from build123d import *

# Parameters (mm, degrees)
F0_W      = 100
F0_H      = 100
F1_DEPTH  = 20
F2_W      = 100
F2_H      = 20
F3_DEPTH  = 80
F4_W      = 30
F4_H      = 80
F5_DEPTH  = 80
F6_SIZE2  = 80
F6_SIZE   = 80
F7_W      = 15
F7_H      = 12.7048021555
F8_DEPTH  = 127
F10_DEPTH = 1143
F11_R     = 15.2311965997
F12_DEPTH = 254
F13_R     = 19.0095175901


with BuildPart() as f1:
    # F0 (on Front) → F1 (new body)
    with BuildSketch(Plane.XZ):
        Rectangle(F0_W, F0_H)
    extrude(amount=F1_DEPTH)

    # F2 (on face) → F3 (join)
    with BuildSketch(Plane.XZ.offset(20)):
        with Locations((0, 40)):
            Rectangle(F2_W, F2_H)
    extrude(amount=F3_DEPTH)

    # F4 (on face) → F5 (join)
    with BuildSketch(Plane.XZ.offset(20)):
        with Locations((35, -10)):
            Rectangle(F4_W, F4_H)
    extrude(amount=F5_DEPTH)

    # F6
    f6_edges = [f1.edges().sort_by_distance(p)[0] for p in [
        (35, -100, -50),
    ]]
    chamfer(f6_edges, length=F6_SIZE, length2=F6_SIZE2)

    # F7 (on face) → F8 (cut)
    with BuildSketch(Plane(origin=(0, 0, 30), x_dir=(1, 0, 0), z_dir=(0, 0, -1))):
        with Locations((-22.5, 66.3524010777)):
            Rectangle(F7_W, F7_H)
        with Locations((-22.5, 53.6475989223)):
            Rectangle(F7_W, F7_H)
        with Locations((-7.5, 53.6475989223)):
            Rectangle(F7_W, F7_H)
        with Locations((-7.5, 66.3524010777)):
            Rectangle(F7_W, F7_H)
    extrude(amount=-F8_DEPTH, mode=Mode.SUBTRACT)

    # F9 (on face) → F10 (cut)
    with BuildSketch(Plane.XZ.offset(20)):
        with BuildLine():
            Line((-25, -25), (-40, -25))
            ThreePointArc((-40, -25), (-35.6066017178, -35.6066017178), (-25, -40))
            Line((-25, -40), (-25, -25))
        make_face()
    extrude(amount=-F10_DEPTH, mode=Mode.SUBTRACT)

    # F11 (on face) → F12 (cut)
    with BuildSketch(Plane.XZ.offset(20)):
        with Locations((-25, -25)):
            Circle(F11_R)
        with BuildLine():
            Line((-40, -25), (-25, -25))
            Line((-25, -25), (-25, -40))
            ThreePointArc((-25, -40), (-35.6066017178, -35.6066017178), (-40, -25))
        make_face(mode=Mode.SUBTRACT)
        with Locations((-25, -25)):
            Circle(F11_R)
    extrude(amount=-F12_DEPTH, mode=Mode.SUBTRACT)

    # F13
    f13_edges = [f1.edges().sort_by_distance(p)[0] for p in [
        (-50, -10, -50),
    ]]
    fillet(f13_edges, radius=F13_R)


solid = f1.part
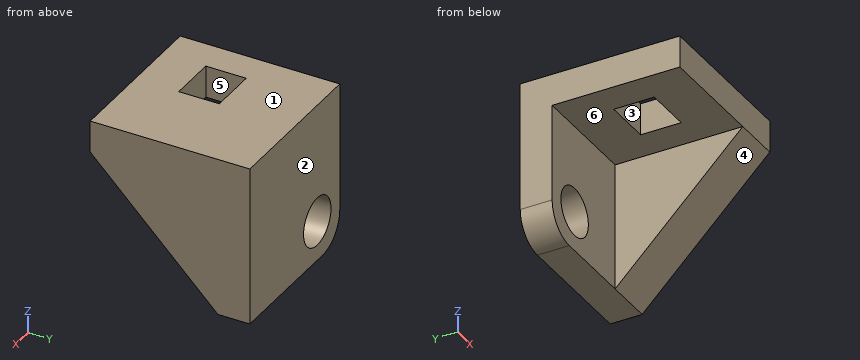
Input: part model. Units: mm. Frame: model coordinates. Face numbers are marked on the shaded views. A direction names the side the tool comes from. Coordinates: 2 decimals unless noted, no trailing zeros. Loops run counter-clockwise (first coordinate to the right, second up) from the corner with the lowest first, then second, coordinate; pieces in that order, holes last. Notation, with made-up numbers: (14.25, 42.25) - (48.25, 42.25) arc R15 cw to (48.25, 62.25) - close; hole circle Ø2 at (-0.75, 80.5). An arc over 180 degrees is marked (long way). Answer in a Markdown table with one row per item. Add a question column.
Item 1: Mould query, pull axis Y, two halves, no side actions, for the marked faces 1, 2 and 3. Classes: released by +Y, released by -Y, zero draft, split by the parting line, or undercut.
Item 2: Contact query for flat-ended pins moving along their axis: P1, Ø21, axis at x = -31.5, z = -29, coming from the -Y side; P2, Ø10, axis at x = 10.5, y = -85.5, coming from the -Z side; P3, Ø24, axis at y = -76.5, z = -9, coming from the -X side. Output: stop coordinate, or through.
Item 3: Section query C-C on x = -25. Return the cut outline in (y, z), then the cut area to 3 significant figures.
Item 4: Section query A-A on z = -25. Return the cut outline in (x, y).
Item 5: Section query B-B on y = -63. Return the cut outline in (x, z), then the cut area to 3 significant figures.
Item 6: Line query: line 1 along Z through (x, y) = (-25, -14); line 2 along Y through (x, z) = (-9, -14); line 3 along Z through (x, y) = (10.5, -23). Output: solid intervals per line, ascending. Write a range as [from, to].
Item 7: Access query for the marked faces 4, 5 and 6. Directions: +Z, -Z, +X, -X, +Y, -Y. A direction counts if a zero-diameter tool reaches every point of the face in a straight line with its end or side. Return the directions, or none.
Item 8: Section query D-D on y = -7. Return the cut outline in (x, z), then the cut area to 3 significant figures.
Recorded:
| question | item | result |
|---|---|---|
| 1 | face 1 | zero draft |
| 1 | face 2 | released by +Y |
| 1 | face 3 | undercut |
| 2 | P1 | y = -20 |
| 2 | P2 | z = 30 |
| 2 | P3 | x = 20 |
| 3 | outline | (-100, 30) - (-72.7, 30) - (-72.7, 50) - (-100, 50) - close; (-47.3, 30) - (-20, 30) - (-20, -9.77) - (0, -9.77) - (0, 50) - (-47.3, 50) - close; (-20, -50) - (0, -50) - (0, -40.23) - (-20, -40.23) - close |
| 3 | area | 2,480 mm^2 |
| 4 | outline | (-50, -20) - (-40.23, -20) - (-40.23, 0) - (-50, 0) - close; (-9.77, -20) - (20, -20) - (20, -45) - (50, -45) - (50, 0) - (-9.77, 0) - close |
| 5 | outline | (-50, 30) - (-30, 30) - (-30, 50) - (-50, 50) - close; (0, 30) - (20, 30) - (20, -7) - (50, -7) - (50, 50) - (0, 50) - close |
| 5 | area | 2,510 mm^2 |
| 6 | line 1 | [-50, -40.23], [-9.77, 50] |
| 6 | line 2 | [-20, 0] |
| 6 | line 3 | [30, 50] |
| 7 | face 4 | -Z, +X, -X, -Y |
| 7 | face 5 | +Z, -Z |
| 7 | face 6 | -Z, -X, -Y |
| 8 | outline | (-50, -30.99) arc R19.01 ccw to (-30.99, -50) - (50, -50) - (50, 50) - (-50, 50) - close; hole circle Ø30.46 at (-25, -25) |
| 8 | area | 9,190 mm^2 |
